```python
from build123d import *

# Parameters (mm, degrees)
F1_DEPTH       = 2.54
F3_DEPTH       = 6.985
F5_D           = 5
F5_CSINK_D     = 9.5
F5_CSINK_ANGLE = 82


with BuildPart() as f1:
    # F0 (on Top) → F1 (new body)
    with BuildSketch(Plane.XY):
        with BuildLine():
            ThreePointArc((10.648604, 20.65796), (5.478705, 22.58601), (0, 23.241))
            Line((0, 23.241), (0, -23.241))
            ThreePointArc((0, -23.241), (5.478705, -22.58601), (10.648604, -20.65796))
            Line((10.648604, -20.65796), (38.241778, -6.434447))
            ThreePointArc((38.241778, -6.434447), (42.164, 0), (38.241778, 6.434447))
            Line((38.241778, 6.434447), (10.648604, 20.65796))
        make_face()
    extrude(amount=F1_DEPTH)

    # F2 (on face) → F3 (join)
    with BuildSketch(Plane(origin=(0, 0, 0), x_dir=(1, 0, 0), z_dir=(0, 0, -1))):
        with BuildLine():
            Line((36.865278, -7.143994), (0, 11.859031))
            Line((0, 11.859031), (0, -23.241))
            ThreePointArc((0, -23.241), (5.478705, -22.58601), (10.648604, -20.65796))
            Line((10.648604, -20.65796), (36.865278, -7.143994))
        make_face()
    extrude(amount=F3_DEPTH)

    # F5 (through all)
    with Locations(Plane.XY.offset(2.54)):
        with Locations((9.525, 3.175)):
            CounterSinkHole(F5_D / 2, F5_CSINK_D / 2, counter_sink_angle=F5_CSINK_ANGLE)


solid = f1.part
```
Could you check a few things on this model? Use its own coordinates, in mm. A direction names the side the tool comes from. Round coordinates to 2 decimals unless told otherwise and drop trailing zeros. Write each loop counter-clockwise with the first axis right and the second up, starting at its lowest first coordinate (ties: lowest second). Pieces come first, ordered by that corner, then holes. Notation, with made-up numbers: M 82,87.5 L 91,87.5 A30 cw 91,125.5 Z; hole C 51,-39.75 d11. An arc over 180 degrees is marked long. Answer in a Markdown table with one row per item. Add a question column.
Q1. Imagine slicing it at A-A (x = 28.5). Please give me the cut outline in (y, z) (3 decimals), then the cut area to 3 significant figures.
Q2. Imagine slicing it at D-D (x = 23.5). Please give me the cut outline in (y, z) (3 decimals), then the cut area to 3 significant figures.
Q3. If I drill on line 1 (Z direction, x = 5, y = -13); line 2 (X direction, y = 3.5, z = -0.5); line 3 (Y direction, x = 30.5, z = -4.5), over which ranges is the centre line in solid material (lowest first)? Write a range as from..to.
Q4. On a 3-axis mill with a long thin cutter (end or side, diameter ignored), from which of +Z, -Z, +X, -X, +Y, -Y can I reach the whole of each face in a straight line? I mean faces 1 (the cylindrical face through (42.163, -0.111, 1.252)), 2 (the flat face through (19, -8, 0)). Say none if no direction works.
Q5. If we mould it in two halves opening along Y, with no side actions, what happens to faces 3 (the flat face through (23.573, 13.996, -3.444)), 4 (the cylindrical face through (11.509, 1.654, -3.565)), 5 (the flat face through (14, 5, -6.985))? For each: +Y half, -Y half, draft (parallel to the pull), parting line (faces both ways), or undercut.
Q6. Imagine slicing it at C-C (z = 1). Please give me the cut outline in (x, y) (3 decimals), then the cut area to 3 significant figures.
Q7. Will these pins go through, and if not, where does the flat tip stop? pin 1 Ø6.5 at (x, y) = (9.525, 3.175) entering from +Z; pin 2 Ø1 at (x, y) = (11, -16.5) entering from -Z; pin 3 Ø4 at (x, z) = (15, 1) entering from -Y.
Q8. Imagine slicing it at B-B (y = 19). Please give me the cut outline in (x, z) (3 decimals), then the cut area to 3 significant figures.
Values:
| question | item | result |
|---|---|---|
| 1 | outline | M -11.456,0 L 2.832,0 L 2.832,-6.985 L 11.456,-6.985 L 11.456,2.54 L -11.456,2.54 Z |
| 1 | area | 118 mm^2 |
| 2 | outline | M -14.033,0 L 0.255,0 L 0.255,-6.985 L 14.033,-6.985 L 14.033,2.54 L -14.033,2.54 Z |
| 2 | area | 168 mm^2 |
| 3 | line 1 | 0..2.54 |
| 3 | line 2 | 0..7.05, 12..29.8 |
| 3 | line 3 | 3.86..10.43 |
| 4 | face 1 | +Z, -Z, +X |
| 4 | face 2 | -Z, +X, -Y |
| 5 | face 3 | +Y half |
| 5 | face 4 | undercut |
| 5 | face 5 | draft |
| 6 | outline | M 0,-23.241 A23.241 ccw 10.649,-20.658 L 38.242,-6.434 A7.239 ccw 38.242,6.434 L 10.649,20.658 A23.241 ccw 0,23.241 Z; hole C 9.525,3.175 d6.823 |
| 6 | area | 1,220 mm^2 |
| 7 | pin 1 | z = 0.81 |
| 7 | pin 2 | z = 0 |
| 7 | pin 3 | y = -19.45 |
| 8 | outline | M 0,-6.985 L 13.865,-6.985 L 13.865,2.54 L 0,2.54 Z |
| 8 | area | 132 mm^2 |
